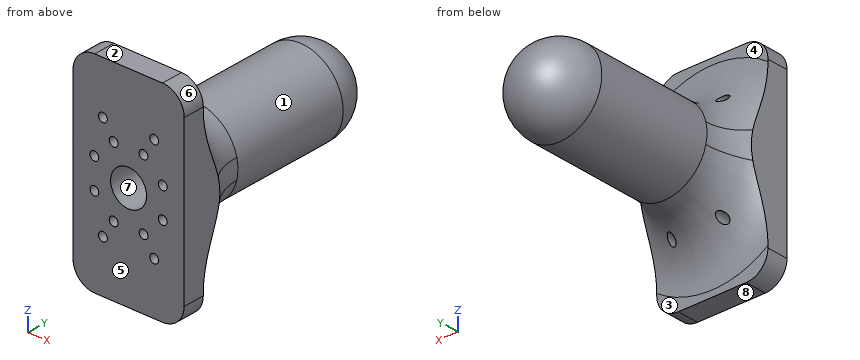
```python
from build123d import *

# Parameters (mm, degrees)
SKETCH1_W                    = 44.069
SKETCH1_H                    = 48.18617301
BOSS_EXTRUDE1_DEPTH          = 5.08
SKETCH2_R                    = 9.9441
BOSS_EXTRUDE2_DEPTH          = 40.64
REVOLVE1_ANGLE               = 180
FILLET1_R                    = 12.7
CUT_EXTRUDE1_DEPTH           = 65.532844704
M2_5X0_45_TAPPED_HOLE1_D     = 2.05
M2_5X0_45_TAPPED_HOLE1_DEPTH = 12
M2_5X0_45_TAPPED_HOLE1_TIP   = 0.615882135
CUT_EXTRUDE2_DEPTH           = 10


with BuildPart() as part:
    # Sketch1 → Boss-Extrude1 (new body)
    with BuildSketch(Plane(origin=(0, 0, 0), x_dir=(1, 0, 0), z_dir=(0, 1, 0))):
        Rectangle(SKETCH1_W, SKETCH1_H)
    extrude(amount=BOSS_EXTRUDE1_DEPTH)

    # Sketch2 → Boss-Extrude2 (add)
    with BuildSketch(Plane(origin=(0, 5.08, 0), x_dir=(1, 0, 0), z_dir=(0, 1, 0))):
        with Locations(Location((0, 0, 0), (0, 0, 270))):
            Circle(SKETCH2_R)
    extrude(amount=BOSS_EXTRUDE2_DEPTH)

    # Sketch3 → Revolve1 (revolve)
    with BuildSketch(Plane(origin=(0, 45.72, 0), x_dir=(1, 0, 0), z_dir=(0, 1, 0))):
        with BuildLine():
            Line((0, 9.9441), (0, -9.9441))
            ThreePointArc((0, -9.9441), (9.9441, 0), (0, 9.9441))
        make_face()
    revolve(axis=Axis((0, 45.72, -9.9441), (0, 0, 1)), revolution_arc=REVOLVE1_ANGLE)

    # Fillet1
    fillet1_edges = [part.edges().sort_by_distance(p)[0] for p in [
        (0, 5.08, -9.9441),
    ]]
    fillet(fillet1_edges, radius=FILLET1_R)

    # Sketch4 → Cut-Extrude1 (cut, through all)
    with BuildSketch(Plane.XZ):
        with BuildLine():
            Line((-22.0345, -24.093086505), (-7.9375, -24.093086505))
            ThreePointArc((-7.9375, -24.093086505), (-11.529602448, -22.605188954), (-13.0175, -19.013086505))
            Line((-13.0175, -19.013086505), (-13.0175, 19.013086505))
            ThreePointArc((-13.0175, 19.013086505), (-11.529602448, 22.605188954), (-7.9375, 24.093086505))
            Line((-7.9375, 24.093086505), (-22.0345, 24.093086505))
            Line((-22.0345, 24.093086505), (-22.0345, -24.093086505))
        make_face()
        with BuildLine():
            ThreePointArc((13.0175, -19.013086505), (11.529602448, -22.605188954), (7.9375, -24.093086505))
            Line((7.9375, -24.093086505), (22.0345, -24.093086505))
            Line((22.0345, -24.093086505), (22.0345, 24.093086505))
            Line((22.0345, 24.093086505), (7.9375, 24.093086505))
            ThreePointArc((7.9375, 24.093086505), (11.529602448, 22.605188954), (13.0175, 19.013086505))
            Line((13.0175, 19.013086505), (13.0175, -19.013086505))
        make_face()
    extrude(amount=-CUT_EXTRUDE1_DEPTH, mode=Mode.SUBTRACT)

    # M2.5x0.45 Tapped Hole1
    with Locations(Plane(origin=(0, 0, 0), x_dir=(-1, 0, 0), z_dir=(0, -1, 0))):
        with Locations((-6.00000248, -11.999988915), (-3.50000248, -7.999988915), (-8.00000248, -3.499988915), (-8.00000248, 3.500011085), (-3.50000248, 8.000011085), (-6.00000248, 12.000011085), (3.49999752, 8.000011085), (5.99999752, 12.000011085), (7.99999752, 3.500011085), (7.99999752, -3.499988915), (3.49999752, -7.999988915), (5.99999752, -11.999988915)):
            Hole(M2_5X0_45_TAPPED_HOLE1_D / 2, depth=M2_5X0_45_TAPPED_HOLE1_DEPTH)
            with Locations((0, 0, -(M2_5X0_45_TAPPED_HOLE1_DEPTH + M2_5X0_45_TAPPED_HOLE1_TIP / 2))):  # 118° drill point
                Cone(0, M2_5X0_45_TAPPED_HOLE1_D / 2, M2_5X0_45_TAPPED_HOLE1_TIP, mode=Mode.SUBTRACT)

    # Sketch5 → Cut-Extrude2 (cut)
    with BuildSketch(Plane.XZ):
        with BuildLine():
            ThreePointArc((2.48e-06, -4.200011085), (4.20000248, -1.1085e-05), (2.48e-06, 4.199988915))
            ThreePointArc((2.48e-06, 4.199988915), (-4.19999752, -1.1085e-05), (2.48e-06, -4.200011085))
        make_face()
    extrude(amount=-CUT_EXTRUDE2_DEPTH, mode=Mode.SUBTRACT)


solid = part.part
```
Work out the finished part from the listing and answer in its coordinate system (mm). Face numbers are marked on the shaded views. A direction names the side the tool comes from. Round coordinates to 2 decimals unless told otherwise and drop trailing zeros. Loops run counter-clockwise (first coordinate to the right, second up) from the corner with the lowest first, then second, coordinate; pieces in that order, holes last.
(1) For the marked faces 1, 2, 3 and 4, determine the directions among +Z, -Z, +X, -X, +Y, -Y from which every point of the face is accessible in a straight line to the end or side of a thin tool.
Computed values:
face 1: +Y
face 2: +Z, +X, -X, +Y, -Y
face 3: -Z, +Y
face 4: +Z, +Y
(2) Find the intervals of material crossed by L1, parallel to X at y = 8, z = 12 (3 decimals); L2, parallel to Z at x = -7, y = 46.5; L3, parallel to Z at x = 1.5, y = 51.5, in increasing order.
Computed values:
L1: x = -8.214 to -7.025, -4.975 to 4.975, 7.025 to 8.214
L2: z = -7.02 to 7.02
L3: z = -7.95 to 7.95
(3) The mould has two halves that part along Z. Classify the marked faces 5, 6, 7 and 8: pulls with the +Z half, pulls with the -Z half, needs draft (parallel to the pull), parting line crosses it, or undercut.
Computed values:
face 5: needs draft
face 6: pulls with the +Z half
face 7: undercut
face 8: pulls with the -Z half
(4) The part is cut by section B-B, the plane y = 47.5. Give the vertices of the cut face in (x, z), and give its area (3 significant figures).
Computed values:
outline: circle Ø19.57 at (0, 0)
area: 301 mm2
(5) The part is cut by section A-A, the plane y = 31. Give the vertices of the cut face in (x, z).
Computed values:
outline: circle Ø19.89 at (0, 0)
(6) Each of these flat-tipped pins is pushed along its axis until it touches: P1, Ø1.8, axis at x = 8, z = -3.5, coming from the -Y side; P2, Ø6, axis at x = 6, z = -21.5, coming from the +Y side; P3, Ø1, axis at y = 39.5, z = -7, coming from the -X side. Where does it stop, or does it pass through?
Computed values:
P1: stops at y = 12.08
P2: stops at y = 5.52
P3: stops at x = -7.53
